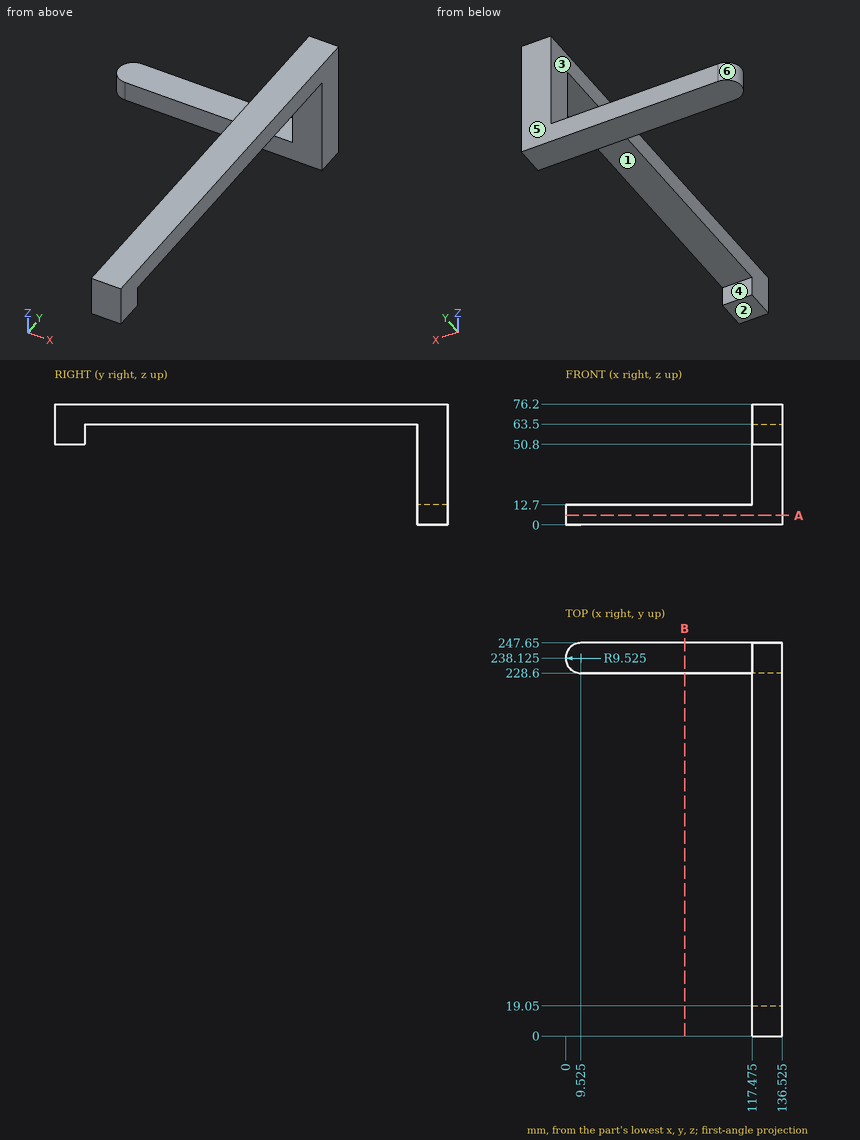
Answer from the drawing. Dimensions are ordinates in mm from the lowest x, y and z of the part. A direction names the side the tool comes from. Give positions to 0.01 mm unless a question says otherwise; leave off trailing zeros. Write each loop counter-clockwise with the first axis right and the second up, starting at its lowest first coordinate (ties: lowest second). Pieces come first, ordered by that corner, then holes. Notation, with made-up numbers: (-39, 32) - (-14, 32) arc R17 cw to (-14, 40) - close; hole circle Ø7 at (42, 87.5). An arc over 180 degrees is marked (long way). One line per item, written item: value. Start each with the question number.
1. Find section B-B (x = 75). Write down the section's boundary in (y, z).
2. For the marked faces 1, 2 and 3, determine the directions among +Z, -Z, +X, -X, +Y, -Y from which every point of the face is accessible in a straight line to the end or side of a thin tool.
3. Given pin 1 (5.5 mm diameter, centred on x = 123.5, y = 172.5, fed in from -Z); pin 2 (5.5 mm diameter, centred on x = 63, y = 242.5, fed in from +Z); pin 3 (9.5 mm diameter, centred on x = 124, y = 6, fed in from -Z), each flat-ended and moving along its own axis, determine where each tip first touches the part or whether it passes through.
4. For a pull along Y with two mould halves and no side action, classify the marked faces 4, 5 and 6 as +Y half, -Y half, draft (parallel to the pull), parting line (faces both ways), or undercut.
5. Consider probe 1 along Y at (x, z) = (129.5, 63); probe 2 along X at (y, z) = (16.5, 67) (3 decimals); probe 3 along Z at (x, y) = (128, 173.5). Determine where each line is inside the solid, lowest interval first.
6. Find section A-A (z = 6). Write down the section's boundary in (x, y) (3 decimals), then the cut area to 3 significant figures.
Geometry results:
1. outline: (228.6, 0) - (247.65, 0) - (247.65, 12.7) - (228.6, 12.7) - close
2. face 1: -Z, +X, -X
2. face 2: -Z, +X, -X, -Y
2. face 3: +Z, -X, +Y, -Y
3. pin 1: z = 63.5
3. pin 2: z = 12.7
3. pin 3: z = 50.8
4. face 4: undercut
4. face 5: +Y half
4. face 6: parting line
5. probe 1: 0 to 19.05, 228.6 to 247.65
5. probe 2: 117.475 to 136.525
5. probe 3: 63.5 to 76.2
6. outline: (9.525, 228.6) - (136.525, 228.6) - (136.525, 247.65) - (9.525, 247.65) arc R9.525 ccw to start
6. area: 2,560 mm2
